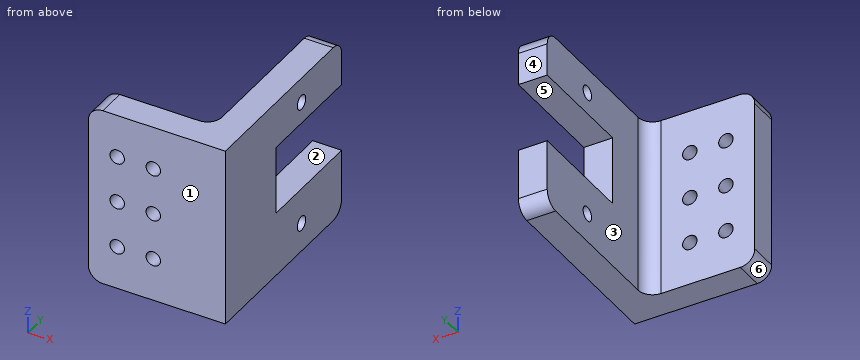
Autodesk Inventor part; units mm, degrees
ref_plane "YZ Plane" through (0, 0, 0) normal (1, 0, 0) x (0, 1, 0)
ref_plane "XZ Plane" through (0, 0, 0) normal (0, 1, 0) x (-1, 0, 0)
ref_plane "XY Plane" through (0, 0, 0) normal (0, 0, 1) x (1, 0, 0)
sketch "Sketch1" plane through (0, 0, 0) normal (0, 1, 0) x (-1, 0, 0)
  line L0 (0, 0) -> (8, 0)
  line L1 (8, 0) -> (8, -50)
  line L2 (8, -50) -> (0, -50)
  line L3 (0, -50) -> (0, 0)
  line L4 (8, 0) -> (38, 0)
  line L5 (38, 0) -> (38, -50)
  line L6 (38, -50) -> (8, -50)
  line L7 (8, -50) -> (8, 0)
  circle A0 centre (30, -12) radius 2
  circle A1 centre (20, -12) radius 2
  circle A2 centre (30, -25) radius 2
  circle A3 centre (20, -25) radius 2
  circle A4 centre (30, -38) radius 2
  circle A5 centre (20, -38) radius 2
  dimension "d15" = 8
  dimension "d16" = 50
  dimension "d17" = 30
extrude "Extrusion3" add sketch "Sketch1" along normal blind 8 contours L4 L5 L6 L1
extrude "Extrusion4" add sketch "Sketch1" along normal blind 55 contours L0 L1 L2 L3
fillet "Fillet1" radius 4 1 edges at (-8, 8, -25)
sketch "Sketch2" plane through (0, 0, 0) normal (1, 0, 0) x (0, 0, -1)
  line L0 (50, 0) -> (0, 0)
  line L1 (10, 8) -> (10, 0)
  circle A0 centre (7, 36) radius 2
  circle A1 centre (42, 36) radius 2
  line L2 (0, 0) -> (0, 55)
  line L3 (50, 0) -> (50, 55)
  line L4 (50, 55) -> (0, 55)
  line L5 (32, 36) -> (32, 24)
  line L6 (32, 24) -> (13, 24)
  line L7 (13, 24) -> (13, 55)
  line L8 (32, 36) -> (32, 55)
  line L9 (13, 55) -> (32, 55)
  dimension "d30" = 7
  dimension "d31" = 50
  dimension "d32" = 35
  dimension "d33" = 8
  dimension "d34" = 18
  dimension "d35" = 19
extrude "Extrusion5" cut sketch "Sketch2" against normal blind 10 contours L8 L5 L6 L7 L4 | A0 | A1
fillet "Fillet2" radius 4 4 edges at (-4, 55, -50) (-4, 55, 0) (-38, 4, 0) (-38, 4, -50)
properties part number "_3DPrint"
Can you work these out from the model? Positions are in its coordinate system, mm. Face numbers are marked on the shaded views. A direction names the side the tool comes from. Coordinates: 2 decimals unless noted, no trailing zeros. Loops run counter-clockwise (first coordinate to the right, second up) from the corner with the lowest first, then second, coordinate; pieces in that order, holes last. Notation, with made-up numbers: M -25,86.25 L -20,86.25 A22 ccw -20,111.25 Z; hole C -8,76 d11. An arc over 180 degrees is marked long. Put each result on its own line as item: value. Start each with the question number.
(1) Imagine slicing it at C-C on y = 43. List the corners of the cut face in (x, z) for me, and give its area (3 significant figures).
(2) Imagine slicing it at B-B on z = -25. List the corners of the cut face in (x, y) for me, and give its area (3 significant figures).
(3) Imagine slicing it at D-D on x = -20. List the corners of the cut face in (y, z) for me.
(4) Which directions (+Z, -Z, +X, -X, +Y, -Y) give clear straight access to the entire face, cutting with the end or side of a thin tool? Please do the marked faces 1, 2 and 3.
(5) We'd pull the mould along Z, two halves only. Please class the marked faces 4, 5 and 6: +Z half, -Z half, draft (parallel to the pull), parting line (faces both ways), or undercut.
(6) Imagine slicing it at A-A on y = 6.5. List the corners of the cut face in (x, z) for me, and give its area (3 significant figures).
(7) I need wall thicknesses on probe 1 along Z at (x, y) = (-30, 4); probe 2 along Z at (x, y) = (-5.5, 39); probe 3 along Y at (x, z) = (-28, -8.5). Which ranges of each line are inside material? Lowest first, please.
(8) Will these pins go through, and if not, where does the flat tip stop? pin 1 Ø2 at (x, z) = (-12, -30.5) entering from -Y; pin 2 Ø6.5 at (x, z) = (-4, -21.5) entering from +Y; pin 3 Ø4.5 at (y, z) = (36, -7) entering from -X; pin 4 Ø13 at (x, z) = (-28, -32) entering from +Y.
Worked answers:
1. outline: M -8,-50 L 0,-50 L 0,-32 L -8,-32 Z; M -8,-13 L 0,-13 L 0,0 L -8,0 Z
1. area: 248 mm2
2. outline: M -38,0 L -32,0 L -32,8 L -38,8 Z; M -28,0 L -22,0 L -22,8 L -28,8 Z; M -18,0 L 0,0 L 0,24 L -8,24 L -8,12 A4 cw -12,8 L -18,8 Z
2. area: 371 mm2
3. outline: M 0,-50 L 8,-50 L 8,-40 L 0,-40 Z; M 0,-36 L 8,-36 L 8,-27 L 0,-27 Z; M 0,-23 L 8,-23 L 8,-14 L 0,-14 Z; M 0,-10 L 8,-10 L 8,0 L 0,0 Z
4. face 1: +Z, -Z, +X, -X, -Y
4. face 2: +X, -X, +Y
4. face 3: +Z, -Z, -X, +Y
5. face 4: draft
5. face 5: undercut
5. face 6: -Z half
6. outline: M -38,-46 A4 ccw -34,-50 L 0,-50 L 0,0 L -34,0 A4 ccw -38,-4 Z; hole C -30,-38 d4; hole C -30,-25 d4; hole C -30,-12 d4; hole C -20,-38 d4; hole C -20,-25 d4; hole C -20,-12 d4
6. area: 1,820 mm2
7. probe 1: z = -50 to -40, -36 to -27, -23 to -14, -10 to 0
7. probe 2: z = -50 to -32, -13 to 0
7. probe 3: y = 0 to 8
8. pin 1: stops at y = 0
8. pin 2: stops at y = 24
8. pin 3: stops at x = -8
8. pin 4: stops at y = 8
